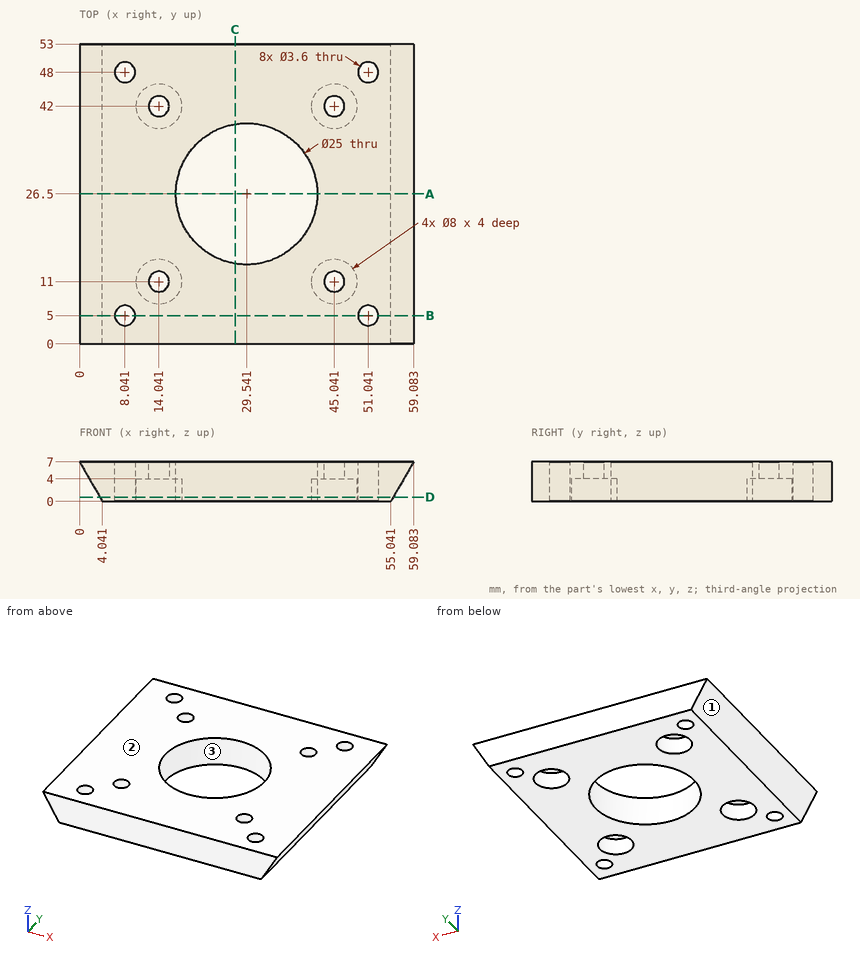
Job drawing, mm, ordinate dimensions from the low corner. One solid piece. Coordinates: 2 decimals unless noted, no trailing zeros. Write each loop counter-clockwise with the first axis right and the second up, starting at its lowest first coordinate (ties: lowest second). Pieces come first, ordered by that corner, then holes.
Item 1: Mould opens along X. For the marked faces 1, 2 and 3 say: released by +X, released by -X, zero draft, split by the parting line, or undercut.
Item 2: Slice it at D-D (z = 0.75). Count the separate pieces of the cut face and the enclosed holes in it, and give its area (3 significant figures).
Item 3: Slice it at C-C (x = 27.5). Write the cut outline in (y, z).
Item 4: Pin check, flat tips, straight feed: pin 1 (6.5 mm diameter, centred on x = 14.04, y = 11, fed in from +Z); pin 2 (6 mm diameter, centred on x = 45.04, y = 42, fed in from -Z). Stop position of each tip, or through.
Item 5: Probe line 1 (Y direction, x = 45, z = 2.75); line 2 (Y direction, x = 51, z = 5.25); line 3 (Y direction, x = 29.5, z = 3.75). List the from-to ranges inside material, lowest first.
Item 6: Slice it at A-A (y = 26.5). Write the cut outline in (x, z).
Item 7: Slice it at B-B (y = 5). Write the cut outline in (x, z), and give its area (3 significant figures).
Results found:
1. face 1: released by -X
1. face 2: zero draft
1. face 3: undercut
2. separate pieces: 1
2. enclosed holes: 9
2. area: 2,020 mm2
3. outline: (0, 0) - (14.17, 0) - (14.17, 7) - (0, 7) - close; (38.83, 0) - (53, 0) - (53, 7) - (38.83, 7) - close
4. pin 1: stops at z = 7
4. pin 2: stops at z = 4
5. line 1: y = 0 to 7, 15 to 38, 46 to 53
5. line 2: y = 0 to 3.2, 6.8 to 46.2, 49.8 to 53
5. line 3: y = 0 to 14, 39 to 53
6. outline: (0, 7) - (4.04, 0) - (17.04, 0) - (17.04, 7) - close; (42.04, 0) - (55.04, 0) - (59.08, 7) - (42.04, 7) - close
7. outline: (0, 7) - (4.04, 0) - (6.24, 0) - (6.24, 7) - close; (9.84, 0) - (49.24, 0) - (49.24, 7) - (9.84, 7) - close; (52.84, 0) - (55.04, 0) - (59.08, 7) - (52.84, 7) - close
7. area: 335 mm2
